Check sheet for the drawn part. Datum: minimum x, y, z corner. Units: mm. Round coordinates to 2 decimals unless told otherwise and drop trailing zeros. Loops run counter-clockwise (first coordinate to the right, second up) from the corner with the lowest first, then second, coordinate; pieces in that order, holes last.
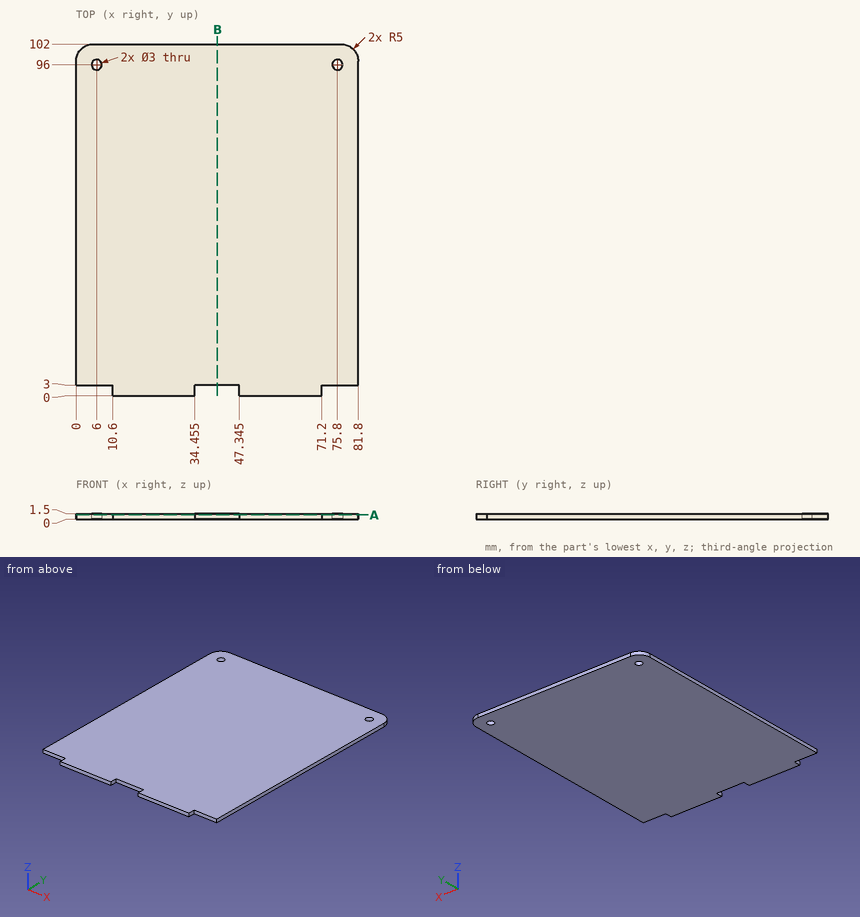
1) Sectioned sample at A-A, the plane z = 1.2. Record the cut outline in (x, y) (3 decimals), then the cut area to 3 significant figures.
Report:
outline: (0, 3) - (10.6, 3) - (10.6, 0) - (34.455, 0) - (34.455, 3) - (47.345, 3) - (47.345, 0) - (71.2, 0) - (71.2, 3) - (81.8, 3) - (81.8, 97) arc R5 ccw to (76.8, 102) - (5, 102) arc R5 ccw to (0, 97) - close; hole circle Ø3 at (6, 96); hole circle Ø3 at (75.8, 96)
area: 8,220 mm2
2) Sectioned sample at B-B, the plane x = 41. Record the cut outline in (y, z), then the cut area to 4 significant figures.
Report:
outline: (3, 0) - (102, 0) - (102, 1.5) - (3, 1.5) - close
area: 148.5 mm2
3) Scan lines: line 1 along X through (y, z) = (96, 0.8); line 2 along Y through (x, z) = (75.8, 0.9); line 3 along Y through (x, z) = (5, 0.45). Record each from-to range of solid material in increasing order.
Report:
line 1: x = 0 to 4.5, 7.5 to 74.3, 77.3 to 81.8
line 2: y = 3 to 94.5, 97.5 to 102
line 3: y = 3 to 94.88, 97.12 to 102
4) Gauge pin test, flat end, axial feed: pin 1 (0.8 mm diameter, centred on y = 1.5, z = 0.5, fed in from -X). Record the tip position at first contact, or that the pin passes through.
Report:
pin 1: stops at x = 10.6
